Check sheet for the modelled part. Datum: model origin and axes. Units: mm. Face numbers are marked on the shaded views. A direction names the side the tool comes from. Give positions to 0.01 mm unless a question says otherwise; leave off trailing zeros. Order: outer loops, then holes, each group sorted by start corner. A loop starts at its lowest first (then second) coordinate and runs counter-clockwise, first axis right, second up.
from build123d import *

# Parameters (mm, degrees)
SALIENTE_EXTRUIR1_DEPTH    = 12
CORTAR_EXTRUIR1_DEPTH      = 31.580715245
CORTAR_EXTRUIR1_DEPTH_BACK = 31.580715245


with BuildPart() as part:
    # Croquis2 → Saliente-Extruir1 (new body)
    with BuildSketch(Plane.XY):
        with BuildLine():
            ThreePointArc((-15.643576177, 12.461080386), (-14.593058293, 10.300539912), (-12.890222435, 8.605879768))
            ThreePointArc((-12.890222435, 8.605879768), (-13.422527733, 7.7495), (-13.898021719, 6.860320205))
            ThreePointArc((-13.898021719, 6.860320205), (-16.217058383, 7.487689244), (-18.613400261, 7.317194183))
            ThreePointArc((-18.613400261, 7.317194183), (-18.793852416, 6.840402867), (-18.962093596, 6.359167119))
            ThreePointArc((-18.962093596, 6.359167119), (-17.23598133, 4.688221457), (-15.056231134, 3.678165989))
            ThreePointArc((-15.056231134, 3.678165989), (-15.263535364, 2.691373106), (-15.406236152, 1.693188893))
            ThreePointArc((-15.406236152, 1.693188893), (-17.799990642, 1.489565697), (-19.993502677, 0.509755553))
            ThreePointArc((-19.993502677, 0.509755553), (-20, 0), (-19.993502677, -0.509755553))
            ThreePointArc((-19.993502677, -0.509755553), (-17.799990642, -1.489565697), (-15.406236152, -1.693188893))
            ThreePointArc((-15.406236152, -1.693188893), (-15.263535364, -2.691373106), (-15.056231134, -3.678165989))
            ThreePointArc((-15.056231134, -3.678165989), (-17.23598133, -4.688221457), (-18.962093596, -6.359167119))
            ThreePointArc((-18.962093596, -6.359167119), (-18.793852416, -6.840402867), (-18.613400261, -7.317194183))
            ThreePointArc((-18.613400261, -7.317194183), (-16.217058383, -7.487689244), (-13.898021719, -6.860320205))
            ThreePointArc((-13.898021719, -6.860320205), (-13.422527733, -7.7495), (-12.890222435, -8.605879768))
            ThreePointArc((-12.890222435, -8.605879768), (-14.593058293, -10.300539912), (-15.643576177, -12.461080386))
            ThreePointArc((-15.643576177, -12.461080386), (-15.320888862, -12.855752194), (-14.98824707, -13.242071204))
            ThreePointArc((-14.98824707, -13.242071204), (-12.678109545, -12.582686962), (-10.713500753, -11.199995653))
            ThreePointArc((-10.713500753, -11.199995653), (-9.962565163, -11.872922824), (-9.16946267, -12.495597438))
            ThreePointArc((-9.16946267, -12.495597438), (-10.189997055, -14.670461235), (-10.438212597, -17.060003452))
            ThreePointArc((-10.438212597, -17.060003452), (-10, -17.320508076), (-9.555290079, -17.569759005))
            ThreePointArc((-9.555290079, -17.569759005), (-7.609993587, -16.160026932), (-6.236773482, -14.188786331))
            ThreePointArc((-6.236773482, -14.188786331), (-5.300970201, -14.56429593), (-4.342730381, -14.878161642))
            ThreePointArc((-4.342730381, -14.878161642), (-4.557871785, -17.270908419), (-3.973846526, -19.601238323))
            ThreePointArc((-3.973846526, -19.601238323), (-3.472963553, -19.69615506), (-2.969824084, -19.778274569))
            ThreePointArc((-2.969824084, -19.778274569), (-1.62400009, -17.788229157), (-1.007799284, -15.466199973))
            ThreePointArc((-1.007799284, -15.466199973), (0, -15.499), (1.007799284, -15.466199973))
            ThreePointArc((1.007799284, -15.466199973), (1.62400009, -17.788229157), (2.969824084, -19.778274569))
            ThreePointArc((2.969824084, -19.778274569), (3.472963553, -19.69615506), (3.973846526, -19.601238323))
            ThreePointArc((3.973846526, -19.601238323), (4.557871785, -17.270908419), (4.342730381, -14.878161642))
            ThreePointArc((4.342730381, -14.878161642), (5.300970201, -14.56429593), (6.236773482, -14.188786331))
            ThreePointArc((6.236773482, -14.188786331), (7.609993587, -16.160026932), (9.555290079, -17.569759005))
            ThreePointArc((9.555290079, -17.569759005), (10, -17.320508076), (10.438212597, -17.060003452))
            ThreePointArc((10.438212597, -17.060003452), (10.189997055, -14.670461235), (9.16946267, -12.495597438))
            ThreePointArc((9.16946267, -12.495597438), (9.962565163, -11.872922824), (10.713500753, -11.199995653))
            ThreePointArc((10.713500753, -11.199995653), (12.678109545, -12.582686962), (14.98824707, -13.242071204))
            ThreePointArc((14.98824707, -13.242071204), (15.320888862, -12.855752194), (15.643576177, -12.461080386))
            ThreePointArc((15.643576177, -12.461080386), (14.593058293, -10.300539912), (12.890222435, -8.605879768))
            ThreePointArc((12.890222435, -8.605879768), (13.422527733, -7.7495), (13.898021719, -6.860320205))
            ThreePointArc((13.898021719, -6.860320205), (16.217058383, -7.487689244), (18.613400261, -7.317194183))
            ThreePointArc((18.613400261, -7.317194183), (18.793852416, -6.840402867), (18.962093596, -6.359167119))
            ThreePointArc((18.962093596, -6.359167119), (17.23598133, -4.688221457), (15.056231134, -3.678165989))
            ThreePointArc((15.056231134, -3.678165989), (15.263535364, -2.691373106), (15.406236152, -1.693188893))
            ThreePointArc((15.406236152, -1.693188893), (17.799990642, -1.489565697), (19.993502677, -0.509755553))
            ThreePointArc((19.993502677, -0.509755553), (20, 0), (19.993502677, 0.509755553))
            ThreePointArc((19.993502677, 0.509755553), (17.799990642, 1.489565697), (15.406236152, 1.693188893))
            ThreePointArc((15.406236152, 1.693188893), (15.263535364, 2.691373106), (15.056231134, 3.678165989))
            ThreePointArc((15.056231134, 3.678165989), (17.23598133, 4.688221457), (18.962093596, 6.359167119))
            ThreePointArc((18.962093596, 6.359167119), (18.793852416, 6.840402867), (18.613400261, 7.317194183))
            ThreePointArc((18.613400261, 7.317194183), (16.217058383, 7.487689244), (13.898021719, 6.860320205))
            ThreePointArc((13.898021719, 6.860320205), (13.422527733, 7.7495), (12.890222435, 8.605879768))
            ThreePointArc((12.890222435, 8.605879768), (14.593058293, 10.300539912), (15.643576177, 12.461080386))
            ThreePointArc((15.643576177, 12.461080386), (15.320888862, 12.855752194), (14.98824707, 13.242071204))
            ThreePointArc((14.98824707, 13.242071204), (12.678109545, 12.582686962), (10.713500753, 11.199995653))
            ThreePointArc((10.713500753, 11.199995653), (9.962565163, 11.872922824), (9.16946267, 12.495597438))
            ThreePointArc((9.16946267, 12.495597438), (10.189997055, 14.670461235), (10.438212597, 17.060003452))
            ThreePointArc((10.438212597, 17.060003452), (10, 17.320508076), (9.555290079, 17.569759005))
            ThreePointArc((9.555290079, 17.569759005), (7.609993587, 16.160026932), (6.236773482, 14.188786331))
            ThreePointArc((6.236773482, 14.188786331), (5.300970201, 14.56429593), (4.342730381, 14.878161642))
            ThreePointArc((4.342730381, 14.878161642), (4.557871785, 17.270908419), (3.973846526, 19.601238323))
            ThreePointArc((3.973846526, 19.601238323), (3.472963553, 19.69615506), (2.969824084, 19.778274569))
            ThreePointArc((2.969824084, 19.778274569), (1.62400009, 17.788229157), (1.007799284, 15.466199973))
            ThreePointArc((1.007799284, 15.466199973), (0, 15.499), (-1.007799284, 15.466199973))
            ThreePointArc((-1.007799284, 15.466199973), (-1.62400009, 17.788229157), (-2.969824084, 19.778274569))
            ThreePointArc((-2.969824084, 19.778274569), (-3.472963553, 19.69615506), (-3.973846526, 19.601238323))
            ThreePointArc((-3.973846526, 19.601238323), (-4.557871785, 17.270908419), (-4.342730381, 14.878161642))
            ThreePointArc((-4.342730381, 14.878161642), (-5.300970201, 14.56429593), (-6.236773482, 14.188786331))
            ThreePointArc((-6.236773482, 14.188786331), (-7.609993587, 16.160026932), (-9.555290079, 17.569759005))
            ThreePointArc((-9.555290079, 17.569759005), (-10, 17.320508076), (-10.438212597, 17.060003452))
            ThreePointArc((-10.438212597, 17.060003452), (-10.189997055, 14.670461235), (-9.16946267, 12.495597438))
            ThreePointArc((-9.16946267, 12.495597438), (-9.962565163, 11.872922824), (-10.713500753, 11.199995653))
            ThreePointArc((-10.713500753, 11.199995653), (-12.678109545, 12.582686962), (-14.98824707, 13.242071204))
            ThreePointArc((-14.98824707, 13.242071204), (-15.320888862, 12.855752194), (-15.643576177, 12.461080386))
        make_face()
    extrude(amount=SALIENTE_EXTRUIR1_DEPTH)

    # Croquis3 → Cortar-Extruir1 (cut, two sides: drawn at the far end of the back side and taken through both)
    with BuildSketch(Plane.XY.offset(12).offset(-CORTAR_EXTRUIR1_DEPTH_BACK)):
        with BuildLine():
            Line((-1.925, -1.74767703), (-1.925, 1.74767703))
            ThreePointArc((-1.925, 1.74767703), (0, 2.6), (1.925, 1.74767703))
            Line((1.925, 1.74767703), (1.925, -1.74767703))
            ThreePointArc((1.925, -1.74767703), (0, -2.6), (-1.925, -1.74767703))
        make_face()
    extrude(amount=CORTAR_EXTRUIR1_DEPTH + CORTAR_EXTRUIR1_DEPTH_BACK, mode=Mode.SUBTRACT)


solid = part.part
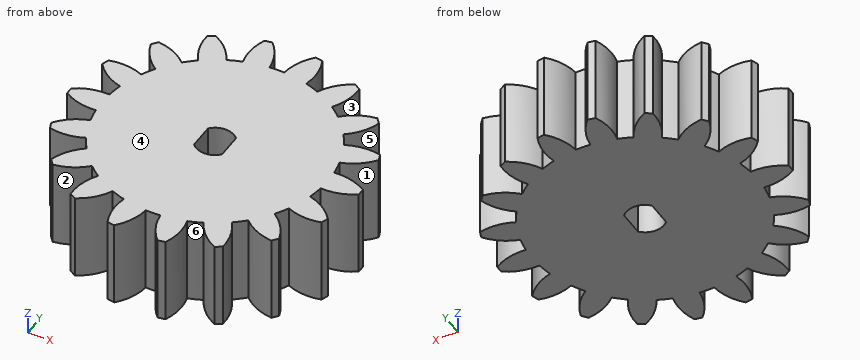
1) Set-up check for the marked faces 1, 2 and 3: record each of +Z, -Z, +X, -X, +Y, -Y from which the full face is reachable in a straight line by a thin tool's end or side.
Recorded:
face 1: +Z, -Z, +X
face 2: +Z, -Z, -Y
face 3: +Z, -Z
2) Material ranges on L1, parallel to Y at x = -13.5, z = 11.75; L2, parallel to Y at x = 15, z = 4; L3, parallel to X at y = 17.5, z = 6.5, recorded low to high.
Recorded:
L1: y = -12.91 to -9.09, -7.61 to 7.61, 9.09 to 12.91
L2: y = -13.23 to -10.94, -7.26 to 7.26, 10.94 to 13.23
L3: x = -9.68 to -9.42, -4.54 to -1.5, 1.5 to 4.54, 9.42 to 9.68
3) Section check B-B, the plane y = 4.5. Record the cut outline in (x, z).
Recorded:
outline: (-16.95, 0) - (16.95, 0) - (16.95, 12) - (-16.95, 12) - close
4) Depth check by flat-ended pin: pin 1 Ø6 at (x, y) = (14, -15) entering from +Z; pin 2 Ø1.5 at (x, z) = (10, 4.5) entering from +Y; pin 3 Ø3 at (x, z) = (-0.5, 6.5) entering from -Y. Enter the tip coordinate at first touch or a pass-through.
Recorded:
pin 1: stops at z = 12
pin 2: stops at y = 17.57
pin 3: stops at y = -18.5
5) Section check A-A, the plane x = 12. Record the cut outline in (y, z), then the cut area to 3 significant figures.
Recorded:
outline: (-12.21, 0) - (12.21, 0) - (12.21, 12) - (-12.21, 12) - close
area: 293 mm2
6) Draft check along X on the marked faces 4, 5 and 6. Enter one of: +X half, -X half, draft (parallel to the pull), parting line (faces both ways), or undercut.
Recorded:
face 4: draft
face 5: +X half
face 6: undercut
